Design review of the part built by this model. Coordinates are the model's own, in mm. A direction names the side the tool comes from. Give positions to 0.01 mm unless a question says otherwise; leave off trailing zeros. Loops run counter-clockwise (first coordinate to the right, second up) from the corner with the lowest first, then second, coordinate; pieces in that order, holes last. Notation, with made-up numbers: (2, 29.5) -> (59, 29.5) arc R20 ccw to (59, 65.5) -> close; hole circle Ø4 at (40.25, 39). An arc over 180 degrees is marked (long way). Answer in a Markdown table with one row per item. Add a question column.
(1) For faces 1 (the flat face through (0, 13.056, -5)), 2 (the cylindrical face through (4.86, 27.253, 0.413)), 3 (the cylindrical face through (-3.35, 6.44, 0.74)), list the 3-axis set-ups (+Z, -Z, +X, -X, +Y, -Y) from which the entire face can be reached by the end or side of a thin tool; tool diameter is ignored.
(2) Consider section A-A on x = 0. Write out the cut boundary in (y, z), then the cut area to 3 significant figures.
(3) Draft analysis for pull direction X (two halves, no side actions). For faces 4 (the flat face through (0, 12, -6.35)), 5 (the flat face through (-3.327, 20, 0)), 6 (the flat face through (-6.35, 15, 0)), 7 (the flat face through (3.327, 20, 0)), state which applies: +X half, -X half, draft (parallel to the pull), parting line (faces both ways), or undercut.
(4) Consider section C-C on y = 13.5. Write out the cut boundary in (x, z).
(5) Consider section D-D on y = 22. Write out the cut boundary in (x, z).
(6) For line 1 (X direction, y = 19, z = -4); line 2 (Y direction, x = 4.85, z = 0); line 3 (Z direction, x = 0, y = 4.75), list the stretches that pass through material, from the lowest coordinate up.
(7) Consider section B-B on z = 0. Write out the cut boundary in (x, y).
(8) For pin 1 (3 mm diameter, centred on x = -1.5, z = -4.5, fed in from +Y), flat-tipped, find the tip position at first contact; note if it passes through.
from build123d import *

# Parameters (mm, degrees)
SKETCH1_W           = 12.7
SKETCH1_H           = 12.7
BOSS_EXTRUDE1_DEPTH = 30.3276
SKETCH2_W           = 6.6548
SKETCH2_H           = 12.7
CUT_EXTRUDE1_DEPTH  = 17.272
SKETCH3_R           = 3.175
CUT_EXTRUDE2_DEPTH  = 34.486950022
SKETCH4_R           = 3.429
CUT_EXTRUDE3_DEPTH  = 13.0556


with BuildPart() as part:
    # Sketch1 → Boss-Extrude1 (new body)
    with BuildSketch(Plane(origin=(0, 0, 0), x_dir=(1, 0, 0), z_dir=(0, 1, 0))):
        Rectangle(SKETCH1_W, SKETCH1_H)
    extrude(amount=BOSS_EXTRUDE1_DEPTH)

    # Sketch2 → Cut-Extrude1 (cut)
    with BuildSketch(Plane(origin=(0, 30.3276, 0), x_dir=(1, 0, 0), z_dir=(0, 1, 0))):
        Rectangle(SKETCH2_W, SKETCH2_H)
    extrude(amount=-CUT_EXTRUDE1_DEPTH, mode=Mode.SUBTRACT)

    # Sketch3 → Cut-Extrude2 (cut, through all)
    with BuildSketch(Plane(origin=(6.35, 0, 0), x_dir=(0, 0, -1), z_dir=(1, 0, 0))):
        with Locations((0, 24.1046)):
            Circle(SKETCH3_R)
    extrude(amount=-CUT_EXTRUDE2_DEPTH, mode=Mode.SUBTRACT)

    # Sketch4 → Cut-Extrude3 (cut)
    with BuildSketch(Plane.XZ):
        with Locations(Location((0, 0, 0), (0, 0, 270))):
            Circle(SKETCH4_R)
    extrude(amount=-CUT_EXTRUDE3_DEPTH, mode=Mode.SUBTRACT)


solid = part.part
Values follow:
| question | item | result |
|---|---|---|
| 1 | face 1 | +Z, -Z, +Y |
| 1 | face 2 | +X, -X |
| 1 | face 3 | -Y |
| 2 | outline | (0, -6.35) -> (13.06, -6.35) -> (13.06, -3.43) -> (0, -3.43) -> close; (0, 3.43) -> (13.06, 3.43) -> (13.06, 6.35) -> (0, 6.35) -> close |
| 2 | area | 76.3 mm2 |
| 3 | face 4 | draft |
| 3 | face 5 | undercut |
| 3 | face 6 | -X half |
| 3 | face 7 | undercut |
| 4 | outline | (-6.35, -6.35) -> (-3.33, -6.35) -> (-3.33, 6.35) -> (-6.35, 6.35) -> close; (3.33, -6.35) -> (6.35, -6.35) -> (6.35, 6.35) -> (3.33, 6.35) -> close |
| 5 | outline | (-6.35, -6.35) -> (-3.33, -6.35) -> (-3.33, -2.38) -> (-6.35, -2.38) -> close; (-6.35, 2.38) -> (-3.33, 2.38) -> (-3.33, 6.35) -> (-6.35, 6.35) -> close; (3.33, -6.35) -> (6.35, -6.35) -> (6.35, -2.38) -> (3.33, -2.38) -> close; (3.33, 2.38) -> (6.35, 2.38) -> (6.35, 6.35) -> (3.33, 6.35) -> close |
| 6 | line 1 | -6.35 to -3.33, 3.33 to 6.35 |
| 6 | line 2 | 0 to 20.93, 27.28 to 30.33 |
| 6 | line 3 | -6.35 to -3.43, 3.43 to 6.35 |
| 7 | outline | (-6.35, 0) -> (-3.43, 0) -> (-3.43, 13.06) -> (-3.33, 13.06) -> (-3.33, 20.93) -> (-6.35, 20.93) -> close; (-6.35, 27.28) -> (-3.33, 27.28) -> (-3.33, 30.33) -> (-6.35, 30.33) -> close; (3.33, 13.06) -> (3.43, 13.06) -> (3.43, 0) -> (6.35, 0) -> (6.35, 20.93) -> (3.33, 20.93) -> close; (3.33, 27.28) -> (6.35, 27.28) -> (6.35, 30.33) -> (3.33, 30.33) -> close |
| 8 | pin 1 | y = 13.06 |
